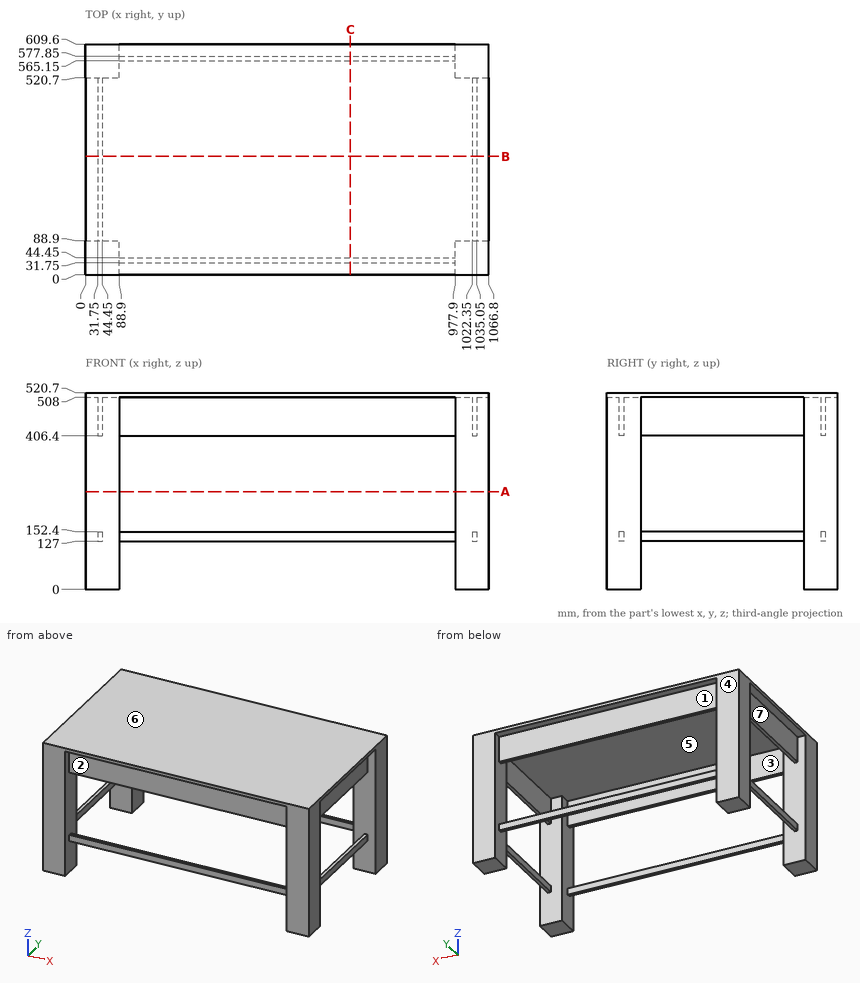
Geometry: see drawing. Coordinates: mm, zero at the bounding-box minimum. A direction names the side the tool comes from. Round coordinates to 2 decimals unless told otherwise and drop trailing zeros. Write each loop counter-clockwise with the first axis right and the second up, starting at its lowest first coordinate (ties: lowest second). Pieces come first, ordered by that corner, then holes. Notation, with made-up numbers: M 6.5,8.25 L 38.5,8.25 A18 ccw 38.5,28.25 Z; hole C -2.75,48.5 d7. An arc over 180 degrees is marked long. Answer as a JSON object with one key per item and string values. Group by question number.
(1) Section query A-A on z = 259. Output: boundary loops of the cut face in (x, y).
(2) Section query B-B on y = 312.5. Output: boundary loops of the cut face in (x, z).
(3) Section query C-C on x = 700.5. Output: boundary loops of the cut face in (y, z), then the cut area to 3 significant figures.
(4) Reachability of the marked faces 1, 2, 3 and 4 from +Z, -Z, +X, -X, +Y, -Y: full face, straight path, thin tool, end or side. Return the list, or none.
(5) Ray query, line 1 (Y direction, x = 76.5, z = 163); line 2 (X direction, y = 196, z = 137); line 3 (Y direction, x = 335, z = 474). Return the intervals inside material, ascending. Write a range as [from, to].
(6) First-contact query: pin 1 (10 mm diameter, centred on x = 38.5, y = 206, fed in from -Z); pin 2 (7.5 mm diameter, centred on y = 250, z = 144, fed in from +X); pin 3 (12.5 mm diameter, centred on x = 731, z = 136.5, fed in from +Y). Flat tips, straight axial feed; report the tip coordinate or a pass-through.
(7) Mould query, pull axis X, two halves, no side actions, for the marked faces 5, 6 and 7. Classes: +X half, -X half, draft (parallel to the pull), parting line (faces both ways), or undercut.
Computed values:
{
 "1": {"outline": "M 0,0 L 88.9,0 L 88.9,88.9 L 0,88.9 Z; M 0,520.7 L 88.9,520.7 L 88.9,609.6 L 0,609.6 Z; M 977.9,0 L 1066.8,0 L 1066.8,88.9 L 977.9,88.9 Z; M 977.9,520.7 L 1066.8,520.7 L 1066.8,609.6 L 977.9,609.6 Z"},
 "2": {"outline": "M 0,508 L 31.75,508 L 31.75,406.4 L 44.45,406.4 L 44.45,508 L 1022.35,508 L 1022.35,406.4 L 1035.05,406.4 L 1035.05,508 L 1066.8,508 L 1066.8,520.7 L 0,520.7 Z; M 31.75,127 L 44.45,127 L 44.45,152.4 L 31.75,152.4 Z; M 1022.35,127 L 1035.05,127 L 1035.05,152.4 L 1022.35,152.4 Z"},
 "3": {"outline": "M 0,508 L 31.75,508 L 31.75,406.4 L 44.45,406.4 L 44.45,508 L 565.15,508 L 565.15,406.4 L 577.85,406.4 L 577.85,508 L 609.6,508 L 609.6,520.7 L 0,520.7 Z; M 31.75,127 L 44.45,127 L 44.45,152.4 L 31.75,152.4 Z; M 565.15,127 L 577.85,127 L 577.85,152.4 L 565.15,152.4 Z", "area": "11,000 mm^2"},
 "4": {"face 1": "-Z, +Y", "face 2": "-Z, -Y", "face 3": "-Z", "face 4": "+Z, -Z, +X, -X, +Y"},
 "5": {"line 1": "[0, 88.9], [520.7, 609.6]", "line 2": "[31.75, 44.45], [1022.35, 1035.05]", "line 3": "[31.75, 44.45], [565.15, 577.85]"},
 "6": {"pin 1": "z = 127", "pin 2": "x = 1035.05", "pin 3": "y = 577.85"},
 "7": {"face 5": "undercut", "face 6": "draft", "face 7": "-X half"}
}
